from build123d import *

# Parameters (mm, degrees)
SKETCH1_W           = 20
SKETCH1_H           = 20
BOSS_EXTRUDE1_DEPTH = 2.5
SKETCH2_W           = 20
SKETCH2_H           = 20
BOSS_EXTRUDE2_DEPTH = 1
SKETCH3_R           = 1.65
CUT_EXTRUDE1_DEPTH  = 4.5


with BuildPart() as part:
    # Sketch1 → Boss-Extrude1 (new body)
    with BuildSketch(Plane.XY):
        Rectangle(SKETCH1_W, SKETCH1_H)
        Polygon((0, -3.210067497), (2.78, -1.605033748), (2.78, 1.605033748), (0, 3.210067497), (-2.78, 1.605033748), (-2.78, -1.605033748), align=None, mode=Mode.SUBTRACT)
    extrude(amount=BOSS_EXTRUDE1_DEPTH)

    # Sketch2 → Boss-Extrude2 (add)
    with BuildSketch(Plane.XY.offset(2.5)):
        Rectangle(SKETCH2_W, SKETCH2_H)
    extrude(amount=BOSS_EXTRUDE2_DEPTH)

    # Sketch3 → Cut-Extrude1 (cut, through all)
    with BuildSketch(Plane(origin=(0, 0, 0), x_dir=(-1, 0, 0), z_dir=(0, 0, -1))):
        Circle(SKETCH3_R)
    extrude(amount=-CUT_EXTRUDE1_DEPTH, mode=Mode.SUBTRACT)


solid = part.part
Geometry: final body of the model. Coordinates: model frame, mm. A direction names the side the tool comes from. Round coordinates to 2 decimals unless told otherwise and drop trailing zeros. Loops run counter-clockwise (first coordinate to the right, second up) from the corner with the lowest first, then second, coordinate; pieces in that order, holes last.
Q1. Pull-direction query (Y, two-part tool) for faces 3 (the flat face through (0, 10, 2)), 4 (the flat face through (-10, 0, 2)), 5 (the flat face through (1.4, 2.4, 1.2)); classes: released by +Y, released by -Y, zero draft, split by the parting line, or undercut.
Q2. Pin query (flat end, axial travel): P1, Ø1.7, axis at x = -0.5, y = -1, coming from the -Z side. Return the tip coordinate at first contact, or that it passes through.
Q3. Section C-C on x = 1. Return loops of the section in (y, z).
Q4. Access query for faces 1 (the flat face through (0, -10, 2)), 2 (the flat face through (-1.4, 2.4, 1.2)). Directions: +Z, -Z, +X, -X, +Y, -Y. A direction counts if a zero-diameter tool reaches every point of the face in a straight line with its end or side. Return the directions, or none.
Q5. Material intervals for L1, parallel to X at y = 0.5, z = 1.15; L2, parallel to Y at x = 0, z = 2.9; L3, parallel to Z at x = 2, y = -1.25, sorted ascending.
Q6. Section B-B on z = 1.25. Return loops of the section in (x, y), plus the area to 3 significant figures.
Q7. Section A-A on y = 0. Return loops of the section in (x, z), plus the area to 3 significant figures.
Q8. Section D-D on y = 2.5. Return loops of the section in (x, z).
Evaluation:
1. face 3: released by +Y
1. face 4: zero draft
1. face 5: undercut
2. P1: stops at z = 2.5
3. outline: (-10, 0) - (-2.63, 0) - (-2.63, 2.5) - (-1.31, 2.5) - (-1.31, 3.5) - (-10, 3.5) - close; (1.31, 2.5) - (2.63, 2.5) - (2.63, 0) - (10, 0) - (10, 3.5) - (1.31, 3.5) - close
4. face 1: +Z, -Z, +X, -X, -Y
4. face 2: -Z
5. L1: x = -10 to -2.78, 2.78 to 10
5. L2: y = -10 to -1.65, 1.65 to 10
5. L3: z = 2.5 to 3.5
6. outline: (-10, -10) - (10, -10) - (10, 10) - (-10, 10) - close; hole (-2.78, -1.61) - (0, -3.21) - (2.78, -1.61) - (2.78, 1.61) - (0, 3.21) - (-2.78, 1.61) - close
6. area: 373 mm2
7. outline: (-10, 0) - (-2.78, 0) - (-2.78, 2.5) - (-1.65, 2.5) - (-1.65, 3.5) - (-10, 3.5) - close; (1.65, 2.5) - (2.78, 2.5) - (2.78, 0) - (10, 0) - (10, 3.5) - (1.65, 3.5) - close
7. area: 52.8 mm2
8. outline: (-10, 0) - (-1.23, 0) - (-1.23, 2.5) - (1.23, 2.5) - (1.23, 0) - (10, 0) - (10, 3.5) - (-10, 3.5) - close
